Design review of the part built by this model. Coordinates are the model's own, in mm. A direction names the side the tool comes from. Give positions to 0.01 mm unless a question says otherwise; leave off trailing zeros. Order: outer loops, then holes, each group sorted by start corner. A loop starts at its lowest first (then second) coordinate and runs counter-clockwise, first axis right, second up. Notation, with made-up numbers: (-35.5, -0.5) -> (-23.5, -0.5) arc R20 cw to (-23.5, 4.5) -> close; hole circle Ø1 at (36.25, -4). An arc over 180 degrees is marked (long way). One line per item, written item: value. Start each with the question number.
1) Tool access review of faces 1 (the face through (0, 0, 0)), 2 (the face through (0.575, 3.18, -1.386)): name each direction out of +Z, -Z, +X, -X, +Y, -Y from which nothing blocks a thin tool from reaching the whole face with its end or side.
2) Consider section A-A (y = 13.25). State the section outline as (x, z) points.
3) Wall thickness on line 1 along Y through (x, z) = (1.05, -1.15); line 2 along X through (y, z) = (10, -2); line 3 along X through (y, z) = (11.75, 1.05): over which ranges is each line inside the solid? List them lowest first. Write a range as from..to.
4) The part is to be moulded in two halves that separate along Z. For faces 3 (the face through (-1, 16, -1)), 4 (the face through (-0.1, 11.1, 2.5)), 5 (the face through (0.27, 12.07, 1.22)), say which applies: released by +Z, released by -Z, zero draft, split by the parting line, or undercut.
5) Consider section C-C (z = 1.9). State the section outline as (x, y) points.
6) For pin 1 (1 mm diameter, centred on x = 1.5, y = 11, fed in from +Z); pin 2 (2.5 mm diameter, centred on x = 0.5, z = 0, fed in from -Y); pin 3 (2 mm diameter, centred on x = 1.5, y = 12, fed in from -Z); pin 4 (1 mm diameter, centred on x = 1, z = 1.5, fed in from -Y), all flat-tipped, find the tip position at first contact; note any pin that passes through.
7) Consider section B-B (y = 3.75). State the section outline as (x, z) points, plus the area to 3 significant figures.
from build123d import *

# Parameters (mm, degrees)
M3_TAPPED_HOLE1_D     = 2.5
M3_TAPPED_HOLE1_DEPTH = 7.748924226
M3_TAPPED_HOLE1_TIP   = 0.751075774


# Read off the part's stored shape, not the designer's step: M3 Machine Threads Stud1
with BuildPart() as part:
    # Sketch2 → Revolve1 (revolve)
    with BuildSketch(Plane.XY, mode=Mode.PRIVATE) as revolve1_sk:
        Polygon((0, 0), (1.5, 0), (1.5, 6), (2.5, 6), (2.5, 16), (0, 16), align=None)
    revolve(revolve1_sk.sketch.rotate(Axis((0, 0, 0), (0, 1, 0)), 90), axis=Axis((0, 0, 0), (0, 1, 0)))

    # M3 Machine Threads Stud1 outline → M3 Machine Threads Stud1 (revolve, cut)
    with BuildSketch(Plane.XY):
        Polygon((1.5, 0.2805), (1.2195, 0), (1.5, 0), align=None)
    revolve(axis=Axis((0, 0, 0), (0, 1, 0)), mode=Mode.SUBTRACT)

    # M3 Tapped Hole1
    with Locations(Plane(origin=(0, 16, 0), x_dir=(1, 0, 0), z_dir=(0, 1, 0))):
        with Locations((0, 0)):
            Hole(M3_TAPPED_HOLE1_D / 2, depth=M3_TAPPED_HOLE1_DEPTH)
            with Locations((0, 0, -(M3_TAPPED_HOLE1_DEPTH + M3_TAPPED_HOLE1_TIP / 2))):  # 118° drill point
                Cone(0, M3_TAPPED_HOLE1_D / 2, M3_TAPPED_HOLE1_TIP, mode=Mode.SUBTRACT)


solid = part.part
Checked values:
1. face 1: +Z, -Z, +X, -X, -Y
1. face 2: -Y
2. outline: circle Ø5 at (0, 0); hole circle Ø2.5 at (0, 0)
3. line 1: y = 6..16
3. line 2: x = -1.5..1.5
3. line 3: x = -2.27..-0.68, 0.68..2.27
4. face 3: zero draft
4. face 4: split by the parting line
4. face 5: undercut
5. outline: (-1.62, 6) -> (1.62, 6) -> (1.62, 16) -> (-1.62, 16) -> close
6. pin 1: stops at z = 2.29
6. pin 2: stops at y = 0
6. pin 3: stops at z = -2.45
6. pin 4: stops at y = 0.08
7. outline: circle Ø3 at (0, 0)
7. area: 7.07 mm^2
